Autodesk Inventor part; units mm, degrees
ref_plane "YZ Plane" through (0, 0, 0) normal (1, 0, 0) x (0, 1, 0)
ref_plane "XZ Plane" through (0, 0, 0) normal (0, 1, 0) x (-1, 0, 0)
ref_plane "XY Plane" through (0, 0, 0) normal (0, 0, 1) x (1, 0, 0)
sketch "Sketch1" plane through (-41, -6, 0) normal (0, 0, -1) x (-1, 0, 0)
  line L0 (-10.2196, -17.8058) -> (-78.2196, -17.8058)
  line L1 (-78.2196, -17.8058) -> (-78.2196, 29.1942)
  line L2 (-78.2196, 29.1942) -> (-10.2196, 29.1942)
  line L3 (-10.2196, 29.1942) -> (-10.2196, -17.8058)
  point P0 (-41, 6)
  dimension "d0" = 68
  dimension "d1" = 47
extrude "Extrusion4" add sketch "Sketch1" along normal blind 30
sketch "Sketch5" plane through (-30.7804, -23.8058, 0) normal (-1, 0, 0) x (0, 0, 1)
  line L0 (0, 47) -> (0, 0)
  line L1 (0, 0) -> (0, 14)
  line L2 (0, 47) -> (0, 33)
  line L3 (0, 14) -> (-11, 14)
  line L4 (-11, 14) -> (-11, 4)
  line L5 (0, 33) -> (-11, 33)
  line L6 (-11, 33) -> (-11, 43)
  line L7 (-11, 4) -> (-24, 4)
  line L8 (-11, 43) -> (-24, 43)
  line L9 (-24, 43) -> (-24, 4)
  line L10 (0, 14) -> (0, 33)
  line L11 (0, 14) -> (0, 0)
  line L12 (0, 0) -> (-30, 0)
  line L13 (-30, 47) -> (-30, 0)
  line L14 (-30, 0) -> (-30, 47)
  line L15 (-30, 47) -> (0, 47)
  line L16 (0, 47) -> (0, 33)
  line L17 (0, 33) -> (0, 47)
  line L18 (-30, 0) -> (0, 0)
  line L19 (0, 0) -> (0, 14)
  line L20 (0, 0) -> (0, 47)
  point P0 (0, 23.8058)
  dimension "d32" = 14
  dimension "d33" = 14
  dimension "d34" = 11
  dimension "d35" = 10
  dimension "d36" = 11
  dimension "d37" = 10
  dimension "d38" = 13
  dimension "d39" = 13
extrude "Extrusion5" cut sketch "Sketch5" against normal blind 68 contours L0 L5 L6 L8 L9 L7 L4 L3 L12 L13 L15
properties part number "Inferior"
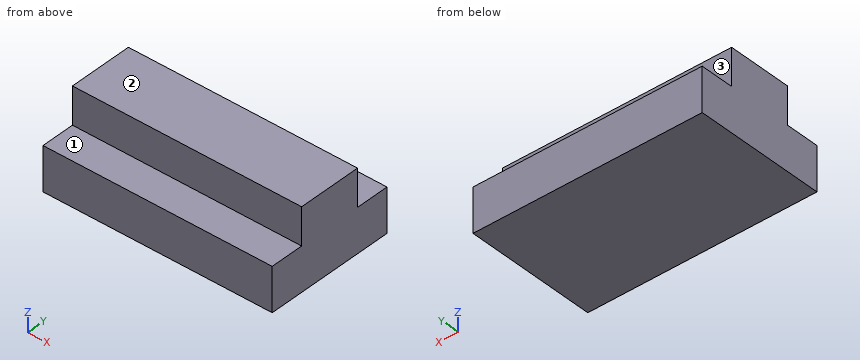
Input: part model. Units: mm. Frame: model coordinates. Face numbers are marked on the shaded views. A direction names the side the tool comes from. Give positions to 0.01 mm unless a question says otherwise; leave off trailing zeros. Order: outer loops, then holes, each group sorted by start corner. A loop starts at its lowest first (then second) coordinate and runs counter-clockwise, first axis right, second up. Notation, with made-up numbers: M -15,-26 L 11,-26 A11 cw 11,-7 Z; hole C 29.25,-11 d3. An arc over 180 degrees is marked long. Answer as a JSON object with one key per item and string values.
1. Reachability of the marked faces 1, 2 and 3 from +Z, -Z, +X, -X, +Y, -Y: full face, straight path, thin tool, end or side. Return the list, or none.
Result sheet:
{"face 1": "+Z, +X, -X, -Y", "face 2": "+Z, +X, -X, +Y, -Y", "face 3": "+Z, +X, -X, +Y"}
2. Ray query, line 1 (Z direction, x = -19, y = 12.5); line 2 (Y direction, x = 17.5, z = -7.25). Return the intervals inside material, ascending. Write a range as [from, to].
Result sheet:
{"line 1": "[-24, -11]", "line 2": "[-9.81, 9.19]"}
3. First-contact query: P1, Ø4, axis at x = 5, z = -7.5, coming from the -Y side; P2, Ø5, axis at x = -4, y = 16.5, coming from the +Z side; P3, Ø12, axis at x = 16, z = -4.5, coming from the +Y side. Flat tips, straight axial feed; report the tip coordinate or a pass-through.
Result sheet:
{"P1": "y = -9.81", "P2": "z = -11", "P3": "y = 9.19"}
4. Cut plane B-B, the plane y = -16. Output: boundary loops of the cut face in (x, z), and give its area (3 significant figures).
Result sheet:
{"outline": "M -30.78,-24 L 37.22,-24 L 37.22,-11 L -30.78,-11 Z", "area": "884 mm²"}
5. Cut plane A-A, the plane x = 5.5. Output: boundary loops of the cut face in (y, z).
Result sheet:
{"outline": "M -19.81,-24 L 19.19,-24 L 19.19,-11 L 9.19,-11 L 9.19,0 L -9.81,0 L -9.81,-11 L -19.81,-11 Z"}
6. Cut plane C-C, the plane z = -5.25. Output: boundary loops of the cut face in (x, y), and give its area (3 significant figures).
Result sheet:
{"outline": "M -30.78,-9.81 L 37.22,-9.81 L 37.22,9.19 L -30.78,9.19 Z", "area": "1,290 mm²"}
